from build123d import *

# Parameters (mm, degrees)
SKETCH1_W               = 0.5
SKETCH1_H               = 3
SKETCH2_R               = 2
BOSS_EXTRUDE1_DEPTH     = 1
SKETCH3_W               = 2.5
SKETCH3_H               = 2
BOSS_EXTRUDE2_DEPTH     = 5
SKETCH4_R               = 1
CUT_EXTRUDE1_DEPTH      = 3
CUT_EXTRUDE1_DEPTH_BACK = 3


with BuildPart() as part:
    # Sketch1 → Revolve1 (revolve)
    with BuildSketch(Plane.XY):
        with Locations((-1.75, 1.5)):
            Rectangle(SKETCH1_W, SKETCH1_H)
    revolve(axis=Axis((0, 0, 0), (0, 1, 0)))

    # Sketch2 → Boss-Extrude1 (add)
    with BuildSketch(Plane(origin=(0, 0, 0), x_dir=(1, 0, 0), z_dir=(0, 1, 0))):
        Circle(SKETCH2_R)
    extrude(amount=-BOSS_EXTRUDE1_DEPTH)

    # Sketch3 → Boss-Extrude2 (add)
    with BuildSketch(Plane.XZ.offset(1)):
        Rectangle(SKETCH3_W, SKETCH3_H)
    extrude(amount=BOSS_EXTRUDE2_DEPTH)

    # Sketch4 → Cut-Extrude1 (cut, two sides)
    with BuildSketch(Plane(origin=(0, 0, 0), x_dir=(-1, 0, 0), z_dir=(0, 0, -1))) as cut_extrude1_sk:
        with Locations((0, -2.973084611)):
            Circle(SKETCH4_R)
    extrude(amount=CUT_EXTRUDE1_DEPTH, mode=Mode.SUBTRACT)
    extrude(cut_extrude1_sk.sketch, amount=-CUT_EXTRUDE1_DEPTH_BACK, mode=Mode.SUBTRACT)


solid = part.part
Model file for the job. Use its own axes, mm. A direction names the side the tool comes from. Give positions to 0.01 mm unless a question says otherwise; leave off trailing zeros. Order: outer loops, then holes, each group sorted by start corner. A loop starts at its lowest first (then second) coordinate and runs counter-clockwise, first axis right, second up. Notation, with made-up numbers: (20, 41) - (41, 41) arc R9 cw to (41, 48) - close; hole circle Ø4 at (83.25, -30.5). An arc over 180 degrees is marked (long way). One line per item, written item: value.
Item 1: Slice it at B-B (z = -0.65). List the corners of the cut face in (x, y).
Response values:
outline: (-1.89, -1) - (-1.25, -1) - (-1.25, -6) - (1.25, -6) - (1.25, -1) - (1.89, -1) - (1.89, 3) - (1.35, 3) - (1.35, 0) - (-1.35, 0) - (-1.35, 3) - (-1.89, 3) - close; hole circle Ø2 at (0, -2.97)
Item 2: Tool access for faces 1 (the flat face through (-1.25, -3, 0)), 2 (the flat face through (0, 0, 0)), 3 (the flat face through (1.25, -3, 0)): list every direction of +Z, -Z, +X, -X, +Y, -Y with a clear straight run to the whole face (end or side of a thin tool).
Response values:
face 1: +Z, -Z, -X, -Y
face 2: +Y
face 3: +Z, -Z, +X, -Y
Item 3: Pin check, flat tips, straight feed: pin 1 Ø1 at (y, z) = (-2.5, 0.5) entering from +X; pin 2 Ø1.5 at (x, z) = (-0.5, 0) entering from +Y; pin 3 Ø1.8 at (x, y) = (0, -2.97) entering from +Z; pin 4 Ø0.6 at (y, z) = (-2.5, 0) entering from -X. Stop position of each tip, or through.
Response values:
pin 1: x = 1.25
pin 2: y = 0
pin 3: through
pin 4: x = -1.25
Item 4: Slice it at C-C (y = -3.5). List the corners of the cut face in (x, z), then the cut area to 3 significant figures.
Response values:
outline: (-1.25, -1) - (-0.85, -1) - (-0.85, 1) - (-1.25, 1) - close; (0.85, -1) - (1.25, -1) - (1.25, 1) - (0.85, 1) - close
area: 1.60 mm2
Item 5: Slice it at D-D (y = 1.5). List the corners of the cut face in (x, z).
Response values:
outline: circle Ø4 at (0, 0); hole circle Ø3 at (0, 0)
Item 6: Wall check: line 1 (Z direction, x = 0, y = 2.05); line 2 (X direction, y = -3, z = 0.2); line 3 (Y direction, x = 0, z = -0.3). Give the ranges that are in metal, low to high.
Response values:
line 1: -2 to -1.5, 1.5 to 2
line 2: -1.25 to -1, 1 to 1.25
line 3: -6 to -3.97, -1.97 to 0
Item 7: Two-plate mould, pull along Z, no slides. Class faces 4 (the flat face through (-1, -4, 1)), 5 (the flat face through (0, -6, 0)), 6 (the flat face through (-1, -4, -1)), 7 (the cylindrical face through (1.5, 1.52, 0.07)): released by +Z, released by -Z, zero draft, split by the parting line, or undercut.
Response values:
face 4: released by +Z
face 5: zero draft
face 6: released by -Z
face 7: undercut
Item 8: Slice it at A-A (x = 0). List the corners of the cut face in (y, z).
Response values:
outline: (-6, -1) - (-3.97, -1) - (-3.97, 1) - (-6, 1) - close; (-1.97, -1) - (-1, -1) - (-1, -2) - (3, -2) - (3, -1.5) - (0, -1.5) - (0, 1.5) - (3, 1.5) - (3, 2) - (-1, 2) - (-1, 1) - (-1.97, 1) - close
